from build123d import *

# Parameters (mm, degrees)
F1_DEPTH  = 3
F2_W      = 22.2
F2_H      = 31
F3_DEPTH  = 25
F4_R      = 13
F5_R      = 13
F6_R      = 5
F7_R      = 5
F8_R      = 5
F9_R      = 5
F10_R     = 2.5
F11_DEPTH = 25
F12_R     = 2.5
F13_DEPTH = 25
F14_R     = 2.5
F15_DEPTH = 25
F16_R     = 2.5
F17_DEPTH = 25


with BuildPart() as f1:
    # F0 (on Front) → F1 (new body)
    with BuildSketch(Plane.XZ):
        Polygon((72.865328, 30), (-57.134672, 30), (-57.134672, -46.7), (36.865328, -46.7), (36.865328, 0), (72.865328, 0), align=None)
    extrude(amount=F1_DEPTH)

    # F2 (on face) → F3 (cut)
    with BuildSketch(Plane.XZ.offset(3)):
        with Locations((-1.734672, -15.5)):
            Rectangle(F2_W, F2_H)
    extrude(amount=-F3_DEPTH, mode=Mode.SUBTRACT)

    # F4
    f4_edges = [f1.edges().sort_by_distance(p)[0] for p in [
        (72.865328, -1.5, 0),
    ]]
    fillet(f4_edges, radius=F4_R)

    # F5
    f5_edges = [f1.edges().sort_by_distance(p)[0] for p in [
        (36.865328, -1.5, 0),
    ]]
    fillet(f5_edges, radius=F5_R)

    # F6
    f6_edges = [f1.edges().sort_by_distance(p)[0] for p in [
        (72.865328, -1.5, 30),
    ]]
    fillet(f6_edges, radius=F6_R)

    # F7
    f7_edges = [f1.edges().sort_by_distance(p)[0] for p in [
        (36.865328, -1.5, -46.7),
    ]]
    fillet(f7_edges, radius=F7_R)

    # F8
    f8_edges = [f1.edges().sort_by_distance(p)[0] for p in [
        (-57.134672, -1.5, -46.7),
    ]]
    fillet(f8_edges, radius=F8_R)

    # F9
    f9_edges = [f1.edges().sort_by_distance(p)[0] for p in [
        (-57.134672, -1.5, 30),
    ]]
    fillet(f9_edges, radius=F9_R)

    # F10 (on face) → F11 (cut)
    with BuildSketch(Plane.XZ.offset(3)):
        with Locations((-52.134672, 25)):
            Circle(F10_R)
    extrude(amount=-F11_DEPTH, mode=Mode.SUBTRACT)

    # F12 (on face) → F13 (cut)
    with BuildSketch(Plane.XZ.offset(3)):
        with Locations((67.865328, 25)):
            Circle(F12_R)
    extrude(amount=-F13_DEPTH, mode=Mode.SUBTRACT)

    # F14 (on face) → F15 (cut)
    with BuildSketch(Plane.XZ.offset(3)):
        with Locations((-52.134672, -41.7)):
            Circle(F14_R)
    extrude(amount=-F15_DEPTH, mode=Mode.SUBTRACT)

    # F16 (on face) → F17 (cut)
    with BuildSketch(Plane.XZ.offset(3)):
        with Locations((31.865328, -41.7)):
            Circle(F16_R)
    extrude(amount=-F17_DEPTH, mode=Mode.SUBTRACT)


solid = f1.part
Build history of the part. All positions in model axes, mm. A direction names the side the tool comes from. Coordinates: 2 decimals unless noted, no trailing zeros. Order: outer loops, then holes, each group sorted by start corner. A loop starts at its lowest first (then second) coordinate and runs counter-clockwise, first axis right, second up. Notation, with made-up numbers: (32, 5) - (65, 5) arc R27 cw to (65, 39) - close; hole circle Ø1 at (16.25, -20). An arc over 180 degrees is marked (long way). Put each result on its own line as item: value.
1. Probe line 1 along X through (y, z) = (-0.95, -18); line 2 along Z through (x, y) = (7, -2.2); line 3 along X through (y, z) = (-0.2, -10.5). List the from-to ranges inside material, lowest first. Write a range as [from, to].
Answer sheet:
line 1: x = [-57.13, -12.83], [9.37, 36.87]
line 2: z = [-46.7, -31], [0, 30]
line 3: x = [-57.13, -12.83], [9.37, 37.11]
2. Saw through at C-C (x = 56). Write the cut outline in (y, z), and give its area (3 significant figures).
Answer sheet:
outline: (-3, 0) - (0, 0) - (0, 30) - (-3, 30) - close
area: 90.0 mm^2
3. Pull direction Z, two halves, no side cores. Call faces 4 (the face through (65.368, -1.521, 25.11)), 5 (the face through (7, 0, 1)), 6 (the face through (-11, -1, -46.7)), 7 (the face through (71.44, -1.521, 28.496)): pulls with the +Z half, pulls with the -Z half, needs draft (parallel to the pull), parting line crosses it, or undercut.
Answer sheet:
face 4: undercut
face 5: needs draft
face 6: pulls with the -Z half
face 7: pulls with the +Z half
4. Saw through at D-D (z = -37). Write the cut outline in (x, y).
Answer sheet:
outline: (-57.13, -3) - (36.87, -3) - (36.87, 0) - (-57.13, 0) - close
5. Saw through at A-A (z = -25.5). Write the cut outline in (x, y).
Answer sheet:
outline: (-57.13, -3) - (-12.83, -3) - (-12.83, 0) - (-57.13, 0) - close; (9.37, -3) - (36.87, -3) - (36.87, 0) - (9.37, 0) - close
6. Drop flat-ended pins along their axis: P1, Ø1.5, axis at y = -1, z = -16, coming from the +X side; P2, Ø1.5, axis at x = 52.5, y = -1.5, coming from the -Z side. Give the stop position or say it passes through.
Answer sheet:
P1: stops at x = 36.87
P2: stops at z = 0
7. Tool access for faces 1 (the face through (72.865, -1, 19)), 2 (the face through (-12.835, -2, -16)), 3 (the face through (36.865, -1, -28)): list every direction of +Z, -Z, +X, -X, +Y, -Y with a clear straight run to the whole face (end or side of a thin tool).
Answer sheet:
face 1: +Z, -Z, +X, +Y, -Y
face 2: +Y, -Y
face 3: -Z, +X, +Y, -Y
8. Saw through at B-B (y = -0.9). Write the cut outline in (x, z).
Answer sheet:
outline: (-57.13, -41.7) arc R5 ccw to (-52.13, -46.7) - (31.87, -46.7) arc R5 ccw to (36.87, -41.7) - (36.87, -13) arc R13 cw to (49.87, 0) - (59.87, 0) arc R13 ccw to (72.87, 13) - (72.87, 25) arc R5 ccw to (67.87, 30) - (-52.13, 30) arc R5 ccw to (-57.13, 25) - close; hole circle Ø5 at (-52.13, -41.7); hole circle Ø5 at (-52.13, 25); hole (-12.83, -31) - (9.37, -31) - (9.37, 0) - (-12.83, 0) - close; hole circle Ø5 at (31.87, -41.7); hole circle Ø5 at (67.87, 25)
